Job drawing, mm, ordinate dimensions from the low corner. One solid piece. A direction names the side the tool comes from. Give positions to 0.01 mm unless a question says otherwise; leave off trailing zeros. Order: outer loops, then holes, each group sorted by start corner. A loop starts at its lowest first (then second) coordinate and runs counter-clockwise, first axis right, second up.
Item 1: Wall check: L1, parallel to Y at x = 4.25, z = 21; L2, parallel to X at y = 1.9, z = 16.51; L3, parallel to X at y = 10.5, z = 14 (1 decimal). Give the ranges that are in metal, low to high.
Item 2: Band-saw the part on B-B on z = 10. Give the cut face in (x, y).
Item 3: Which spindle directions (+Z, -Z, +X, -X, +Y, -Y) get a long thin tool onto all of the face, cutting with end or side? Do the marked faces 5, 6 and 7. Say none if no direction does.
Item 4: Band-saw the part on A-A on y = 6.35. Give the cut face in (x, z) (1 decimal).
Item 5: Two-plate mould, pull along Y, no slides. Class the marked faces 1, 2, 3 and 4: released by +Y, released by -Y, zero draft, split by the parting line, or undercut.
Item 6: Flat gauge pin, fed straight in: P1, Ø5.5, axis at x = 8, y = 5, coming from the +Z side. Where does the tip first touch, or does it go through?
Item 7: Band-saw the part on C-C on z = 16.51. Give the cut face in (x, y).
Item 8: Band-saw the part on D-D on x = 8. Give the cut face in (y, z) (1 decimal), plus the area to 3 significant figures.
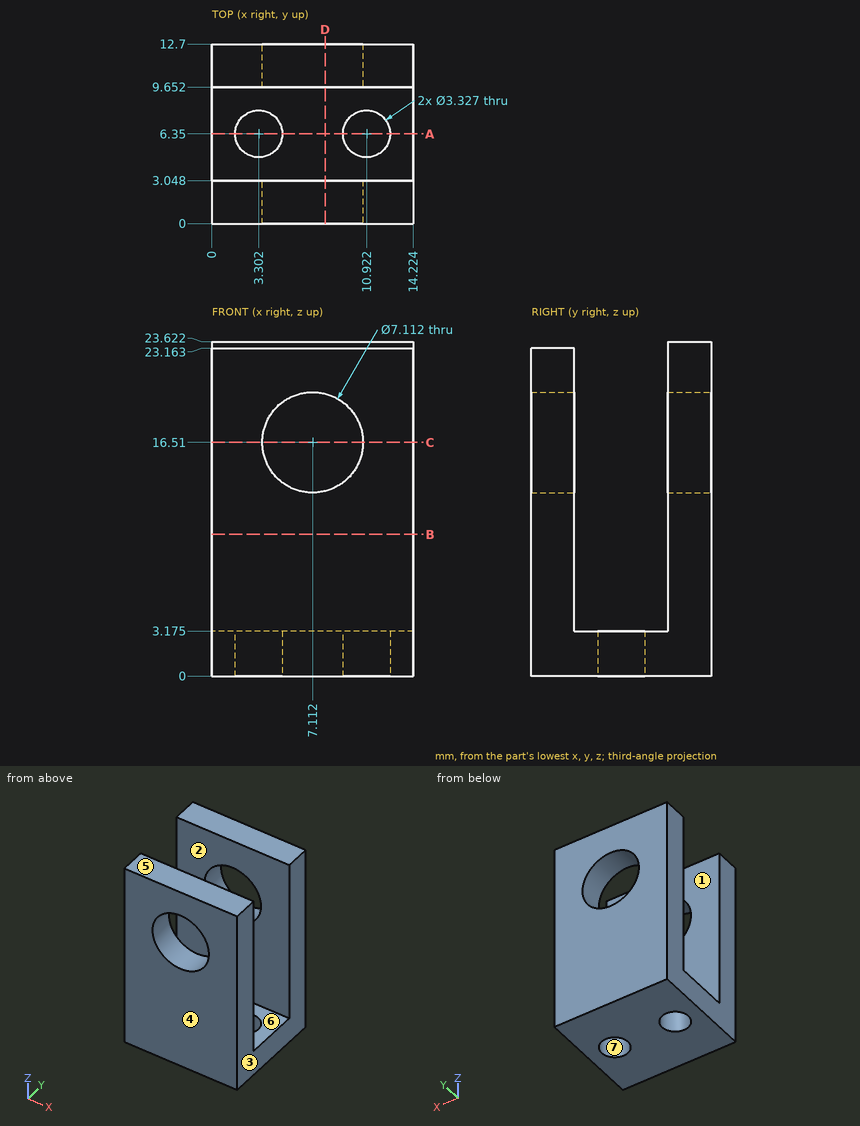
The answers:
1. L1: y = 0 to 3.05, 9.65 to 12.7
1. L2: x = 0 to 3.56, 10.67 to 14.22
1. L3: x = 0 to 4.6, 9.6 to 14.2
2. outline: (0, 0) - (14.22, 0) - (14.22, 3.05) - (0, 3.05) - close; (0, 9.65) - (14.22, 9.65) - (14.22, 12.7) - (0, 12.7) - close
3. face 5: +Z, +X, -X, -Y
3. face 6: +Z, +X, -X
3. face 7: +Z, -Z
4. outline: (0, 0) - (1.6, 0) - (1.6, 3.2) - (0, 3.2) - close; (5, 0) - (9.3, 0) - (9.3, 3.2) - (5, 3.2) - close; (12.6, 0) - (14.2, 0) - (14.2, 3.2) - (12.6, 3.2) - close
5. face 1: undercut
5. face 2: undercut
5. face 3: zero draft
5. face 4: released by -Y
6. P1: stops at z = 23.16
7. outline: (0, 0) - (3.56, 0) - (3.56, 3.05) - (0, 3.05) - close; (0, 9.65) - (3.56, 9.65) - (3.56, 12.7) - (0, 12.7) - close; (10.67, 0) - (14.22, 0) - (14.22, 3.05) - (10.67, 3.05) - close; (10.67, 9.65) - (14.22, 9.65) - (14.22, 12.7) - (10.67, 12.7) - close
8. outline: (0, 0) - (12.7, 0) - (12.7, 13.1) - (9.7, 13.1) - (9.7, 3.2) - (3, 3.2) - (3, 13.1) - (0, 13.1) - close; (0, 20) - (3, 20) - (3, 23.2) - (0, 23.2) - close; (9.7, 20) - (12.7, 20) - (12.7, 23.6) - (9.7, 23.6) - close
8. area: 122 mm2
